```python
from build123d import *

# Parameters (mm, degrees)
BOSS_EXTRUDE1_DEPTH = 2.4
FILLET1_R           = 4
FILLET2_R           = 4
FILLET3_R           = 2


with BuildPart() as part:
    # Sketch1 → Boss-Extrude1 (new body)
    with BuildSketch(Plane(origin=(0, 0, 0), x_dir=(1, 0, 0), z_dir=(0, 1, 0))):
        Polygon((-11, -15), (11, -15), (11, 15), (-11, 15), (-11, -1.3), (-2.5, -1.3), (-2.5, 10), (2.5, 10), (2.5, -6.5), (-2.5, -6.5), (-11, -6.5), align=None)
    extrude(amount=BOSS_EXTRUDE1_DEPTH)

    # Fillet1
    fillet1_edges = [part.edges().sort_by_distance(p)[0] for p in [
        (-2.5, 1.2, 1.3),
    ]]
    fillet(fillet1_edges, radius=FILLET1_R)

    # Fillet2
    fillet2_edges = [part.edges().sort_by_distance(p)[0] for p in [
        (11, 1.2, 15),
        (-11, 1.2, 15),
        (-11, 1.2, -15),
        (11, 1.2, -15),
    ]]
    fillet(fillet2_edges, radius=FILLET2_R)

    # Fillet3
    fillet3_edges = [part.edges().sort_by_distance(p)[0] for p in [
        (-11, 1.2, 6.5),
        (2.5, 1.2, 6.5),
        (-11, 1.2, 1.3),
    ]]
    fillet(fillet3_edges, radius=FILLET3_R)


solid = part.part
```
Input: part model. Units: mm. Frame: model coordinates. A direction names the side the tool comes from. Round coordinates to 2 decimals unless told otherwise and drop trailing zeros. Loops run counter-clockwise (first coordinate to the right, second up) from the corner with the lowest first, then second, coordinate; pieces in that order, holes last. Notation, with made-up numbers: (-12.5, 18) - (-6.5, 18) arc R26 cw to (-6.5, 41) - close; hole circle Ø10 at (54.25, 57). An arc over 180 degrees is marked (long way). One line per item, written item: value. Start each with the question number.
(1) Section A-A, the plane z = -9. Return loops of the section in (x, y).
(2) Section D-D, the plane z = 2.5. Return loops of the section in (x, y), plus the area to 3 significant figures.
(3) Access query for faces 4 (the flat face through (-2.5, 1, -6)), 5 (the cylindrical face through (9.797, 1.217, -13.859)), 6 (the cylindrical face through (1.93, 1.22, 5.9)). Directions: +Z, -Z, +X, -X, +Y, -Y. A direction counts if a zero-diameter tool reaches every point of the face in a straight line with its end or side. Return the directions, or none.
(4) Ray query, line 1 (X direction, y = 1.55, z = -6.5); line 2 (Z direction, x = 0, y = 0.55); line 3 (X direction, y = 2.15, z = 0). Return the intervals inside material, ascending. Write a range as [from, to].
(5) Section C-C, the plane y = 0.95. Return loops of the section in (x, z).
(6) Draft query along X for faces 1 (the cylindrical face through (-10.4, 1.22, 7.07)), 2 (the flat face through (-3, 2.4, -4)), 3 (the flat face through (0, 1, -10)). Return one class per face: +X half, -X half, draft (parallel to the pull), parting line (faces both ways), or undercut.
(7) Contact query for a flat-ended pin moving along its axis: P1, Ø4, axis at x = -1.5, z = 4, coming from the +Y side. Output: stop coordinate, or through.
(8) Section B-B, the plane x = -0.5. Return loops of the section in (y, z), plus the area to 3 significant figures.
Results below:
1. outline: (-11, 0) - (-2.5, 0) - (-2.5, 2.4) - (-11, 2.4) - close; (2.5, 0) - (11, 0) - (11, 2.4) - (2.5, 2.4) - close
2. outline: (2.5, 0) - (11, 0) - (11, 2.4) - (2.5, 2.4) - close
2. area: 20.4 mm^2
3. face 4: +Y, -Y
3. face 5: -Z, +X, +Y, -Y
3. face 6: -X, +Y, -Y
4. line 1: [-11, -2.5], [2.5, 11]
4. line 2: [-15, -10], [6.5, 15]
4. line 3: [-10.87, -3.55], [2.5, 11]
5. outline: (-11, -11) arc R4 ccw to (-7, -15) - (7, -15) arc R4 ccw to (11, -11) - (11, 11) arc R4 ccw to (7, 15) - (-7, 15) arc R4 ccw to (-11, 11) - (-11, 8.5) arc R2 ccw to (-9, 6.5) - (0.5, 6.5) arc R2 cw to (2.5, 4.5) - (2.5, -10) - (-2.5, -10) - (-2.5, -2.7) arc R4 ccw to (-6.5, 1.3) - (-9, 1.3) arc R2 ccw to (-11, -0.7) - close
6. face 1: -X half
6. face 2: draft
6. face 3: undercut
7. P1: through
8. outline: (0, -15) - (2.4, -15) - (2.4, -10) - (0, -10) - close; (0, 6.5) - (2.4, 6.5) - (2.4, 15) - (0, 15) - close
8. area: 32.4 mm^2
